```python
from build123d import *

# Parameters (mm, degrees)
SKETCH1_W                       = 25.4
SKETCH1_H                       = 25.4
SKETCH1_W_2                     = 22.225
SKETCH1_H_2                     = 22.225
BOSS_EXTRUDE1_DEPTH             = 228.6
SKETCH2_R                       = 3.175
CUT_EXTRUDE1_DEPTH              = 231.35713577
SKETCH3_R                       = 3.175
CUT_EXTRUDE2_DEPTH              = 231.35713577
CUT_EXTRUDE3_DEPTH              = 231.35713577
SKETCH6_W                       = 25.4
SKETCH6_H                       = 25.4
SKETCH6_W_2                     = 22.225
SKETCH6_H_2                     = 22.225
BOSS_EXTRUDE3_DEPTH             = 279.4
BOSS_EXTRUDE3_DIRECTION_2_REACH = 232.357


with BuildPart() as part:
    # Sketch1 → Boss-Extrude1 (new body)
    with BuildSketch(Plane(origin=(0, 0, 0), x_dir=(1, 0, 0), z_dir=(0, 1, 0))):
        Rectangle(SKETCH1_W, SKETCH1_H)
        Rectangle(SKETCH1_W_2, SKETCH1_H_2, mode=Mode.SUBTRACT)
    extrude(amount=BOSS_EXTRUDE1_DEPTH)

    # Sketch2 → Cut-Extrude1 (cut, through all)
    with BuildSketch(Plane(origin=(12.7, 0, 0), x_dir=(0, 0, -1), z_dir=(1, 0, 0))):
        with Locations((0, 215.9)):
            Circle(SKETCH2_R)
        with Locations((0, 165.1)):
            Circle(SKETCH2_R)
    extrude(amount=-CUT_EXTRUDE1_DEPTH, mode=Mode.SUBTRACT)

    # Sketch3 → Cut-Extrude2 (cut, through all)
    with BuildSketch(Plane.XY.offset(12.7)):
        with Locations((0, 69.85)):
            Circle(SKETCH3_R)
        with Locations((0, 19.05)):
            Circle(SKETCH3_R)
    extrude(amount=-CUT_EXTRUDE2_DEPTH, mode=Mode.SUBTRACT)

    # Sketch4 → Cut-Extrude3 (cut, through all)
    with BuildSketch(Plane.XY.offset(12.7)):
        Polygon((-12.7, 0), (-12.7, 108.6), (12.7, 134), (12.7, 0), align=None)
    extrude(amount=-CUT_EXTRUDE3_DEPTH, mode=Mode.SUBTRACT)

    # Sketch6 → Boss-Extrude3 (add)
    with BuildSketch(Plane(origin=(12.7, 0, 0), x_dir=(0, 0, -1), z_dir=(1, 0, 0))):
        with Locations((0, 121.3)):
            Rectangle(SKETCH6_W, SKETCH6_H)
        with Locations((0, 121.3)):
            Rectangle(SKETCH6_W_2, SKETCH6_H_2, mode=Mode.SUBTRACT)
    extrude(amount=BOSS_EXTRUDE3_DEPTH)

    # Sketch6 → Boss-Extrude3 direction 2 (add, up to next)
    with BuildSketch(Plane(origin=(12.7, 0, 0), x_dir=(0, 0, -1), z_dir=(1, 0, 0)), mode=Mode.PRIVATE) as boss_extrude3_direction_2_sk1:
        with Locations((0, 121.3)):
            Rectangle(SKETCH6_W, SKETCH6_H)
        with Locations((0, 121.3)):
            Rectangle(SKETCH6_W_2, SKETCH6_H_2, mode=Mode.SUBTRACT)
    boss_extrude3_direction_2_tool1 = extrude(boss_extrude3_direction_2_sk1.sketch, amount=-BOSS_EXTRUDE3_DIRECTION_2_REACH, mode=Mode.PRIVATE) - part.part
    add(boss_extrude3_direction_2_tool1.solids().sort_by_distance((12.7, 121.3, 12.34079))[0])


solid = part.part
```
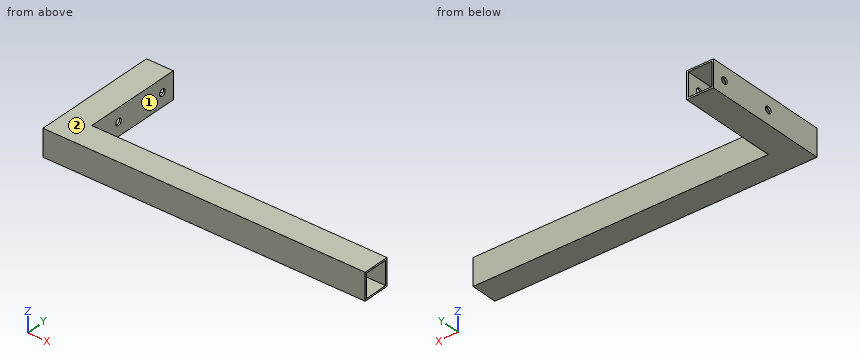
Could you check a few things on this model? Use its own coordinates, in mm. Face numbers are marked on the shaded views. A direction names the side the tool comes from. Round coordinates to 2 decimals unless told otherwise and drop trailing zeros. Loops run counter-clockwise (first coordinate to the right, second up) from the corner with the lowest first, then second, coordinate; pieces in that order, holes last. Notation, with made-up numbers: (5, 45.5) -> (59, 45.5) arc R30 cw to (59, 79.5) -> close; hole circle Ø11 at (-4.5, 16). An arc over 180 degrees is marked (long way). One line per question, with ' | ' between items.
(1) For the marked faces 1 and 2, which set-ups out of +Z, -Z, +X, -X, +Y, -Y let a thin tool reach every point of the face, with its end or its side?
Model answer:
face 1: +Z, -Z, +X, +Y | face 2: +Z, +X, -X, +Y, -Y
(2) If we section it at C-C on x = 36: List the corners of the cut face in (y, z) for me, and give its area (3 significant figures).
Model answer:
outline: (108.6, -12.7) -> (134, -12.7) -> (134, 12.7) -> (108.6, 12.7) -> close; hole (110.19, -11.11) -> (132.41, -11.11) -> (132.41, 11.11) -> (110.19, 11.11) -> close | area: 151 mm^2
(3) If we section it at D-D on y = 120: List the corners of the cut face in (x, z) for me.
Model answer:
outline: (-12.7, -12.7) -> (292.1, -12.7) -> (292.1, -11.11) -> (-11.11, -11.11) -> (-11.11, 11.11) -> (292.1, 11.11) -> (292.1, 12.7) -> (-12.7, 12.7) -> close
(4) If we section it at A-A on y = 215.9: List the corners of the cut face in (x, z) for me (1 decimal), and give its area (3 significant figures).
Model answer:
outline: (-12.7, -12.7) -> (12.7, -12.7) -> (12.7, -3.2) -> (11.1, -3.2) -> (11.1, -11.1) -> (-11.1, -11.1) -> (-11.1, -3.2) -> (-12.7, -3.2) -> close; (-12.7, 3.2) -> (-11.1, 3.2) -> (-11.1, 11.1) -> (11.1, 11.1) -> (11.1, 3.2) -> (12.7, 3.2) -> (12.7, 12.7) -> (-12.7, 12.7) -> close | area: 131 mm^2
(5) If I drill on probe 1 along Y at (x, z) = (-11.9, 0) (3 decimals); probe 2 along Y at (x, z) = (11.6, 0) (1 decimal); probe 3 along Z at (x, y) = (12, 165), over which ranges is the centre line in solid material (lowest first)?
Model answer:
probe 1: y = 108.6 to 161.925, 168.275 to 212.725, 219.075 to 228.6 | probe 2: y = 108.6 to 110.2, 132.4 to 161.9, 168.3 to 212.7, 219.1 to 228.6 | probe 3: z = -12.7 to -3.17, 3.17 to 12.7
(6) If we section it at B-B on z = 6.25: List the corners of the cut face in (x, y) for me.
Model answer:
outline: (-12.7, 108.6) -> (292.1, 108.6) -> (292.1, 110.19) -> (-11.11, 110.19) -> (-11.11, 228.6) -> (-12.7, 228.6) -> close; (11.11, 132.41) -> (292.1, 132.41) -> (292.1, 134) -> (12.7, 134) -> (12.7, 228.6) -> (11.11, 228.6) -> close
(7) For pin 1 Ø11 at (y, z) = (156, -5) entering from +X; pin 2 Ø5 at (y, z) = (215.9, 0) entering from -X; pin 3 Ø4 at (x, z) = (200, 5.5) entering from +Y, each with a flat end and sliding along its axis, tell me the tip position at first contact or that it passes through.
Model answer:
pin 1: stops at x = 12.7 | pin 2: passes through | pin 3: stops at y = 134
